Geometry check sheet. Reference: the model listing, model coordinates, mm. A direction names the side the tool comes from. Round coordinates to 2 decimals unless told otherwise and drop trailing zeros. Loops run counter-clockwise (first coordinate to the right, second up) from the corner with the lowest first, then second, coordinate; pieces in that order, holes last. Notation, with made-up numbers: (17, -5) -> (76, -5) arc R29 cw to (76, 32) -> close; hole circle Ø11 at (45.25, 12.25). An arc over 180 degrees is marked (long way). Use a Markdown table: item, result. Add a question column.
Q1. Material ranges on L1, parallel to Y at x = 5, z = -6; L2, parallel to Z at x = 50, y = 2; L3, parallel to X at y = -1.75, z = 4, recorded low to high.
Q2. Gauge pin test, flat ends, axial feed: P1, Ø4, axis at x = 39.5, y = 8.5, coming from the +Z side; P2, Ø12, axis at x = 51.5, z = 20, coming from the -Y side; P3, Ø5, axis at y = 4, z = 0, coming from the +X side. Record the tip position at first contact, or that the pin passes through.
Q3. Sectioned sample at C-C, the plane y = -3.25. Enter the section's corners in (x, z).
Q4. Release check for a two-part mould opening along X. For faces 1 (the face through (0, -5, 0)), 2 (the face through (47.88, 4.93, 7.16)), 3 (the face through (56.97, 4.93, 1.58)) record: released by +X, released by -X, zero draft, split by the parting line, or undercut.
Q5. Set-up check for faces 4 (the face through (43.989, 4.93, 59.955)), 5 (the face through (2.018, -2.465, 4.868)): record each of +Z, -Z, +X, -X, +Y, -Y from which the full face is reachable in a straight line by a thin tool's end or side.
Q6. Sectioned sample at D-D, the plane z = 9. Enter the section's corners in (x, y), then the cut area to 3 significant figures.
```python
from build123d import *

# Parameters (mm, degrees)
BOSS_EXTRUDE2_DEPTH = 10
SKETCH5_R           = 5.271415538
BOSS_EXTRUDE3_DEPTH = 5
SKETCH8_R           = 5.27
BOSS_EXTRUDE4_DEPTH = 5


with BuildPart() as part:
    # Sketch4 → Boss-Extrude2 (new body)
    with BuildSketch(Plane(origin=(0, 0, 0), x_dir=(1, 0, 0), z_dir=(0, 1, 0))):
        with BuildLine():
            ThreePointArc((51.493202039, -60.650498275), (56.375212409, -0.863559663), (-3.411726203, 4.018450707))
            ThreePointArc((-3.411726203, 4.018450707), (-4.018450707, -3.411726203), (3.411726203, -4.018450707))
            ThreePointArc((3.411726203, -4.018450707), (48.338310994, -7.687012068), (44.669749634, -52.61359686))
            ThreePointArc((44.669749634, -52.61359686), (44.063025129, -60.04377377), (51.493202039, -60.650498275))
        make_face()
    extrude(amount=BOSS_EXTRUDE2_DEPTH)

    # Sketch5 → Boss-Extrude3 (add)
    with BuildSketch(Plane(origin=(0, 10, 0), x_dir=(1, 0, 0), z_dir=(0, 1, 0))):
        with Locations(Location((0, 0, 0), (0, 0, 130.331767004))):
            Circle(SKETCH5_R)
    extrude(amount=BOSS_EXTRUDE3_DEPTH)

    # Sketch8 → Boss-Extrude4 (add)
    with BuildSketch(Plane.XZ):
        with Locations(Location((0, 0, 0), (0, 0, 90))):
            Circle(SKETCH8_R)
    extrude(amount=BOSS_EXTRUDE4_DEPTH)


solid = part.part
```
Values:
| question | item | result |
|---|---|---|
| 1 | L1 | 0 to 10 |
| 1 | L2 | -5.23 to 9.82, 46.81 to 61.54 |
| 1 | L3 | -3.43 to 3.43 |
| 2 | P1 | z = 1.65 |
| 2 | P2 | y = 0 |
| 2 | P3 | x = 57.7 |
| 3 | outline | circle Ø10.54 at (0, 0) |
| 4 | face 1 | zero draft |
| 4 | face 2 | undercut |
| 4 | face 3 | split by the parting line |
| 5 | face 4 | +Y, -Y |
| 5 | face 5 | -Y |
| 6 | outline | (49.39, 0) -> (61.8, 0) -> (61.8, 10) -> (49.39, 10) -> close |
| 6 | area | 124 mm^2 |
